Source: CAD feature listing. Evaluate the final solid. Frame: model axes, mm. A direction names the side the tool comes from. Round coordinates to 2 decimals unless told otherwise and drop trailing zeros. Loops run counter-clockwise (first coordinate to the right, second up) from the corner with the lowest first, then second, coordinate; pieces in that order, holes last. Notation, with made-up numbers: M 83,60.5 L 135,60.5 A7 cw 135,64.5 Z; hole C 32.25,42.5 d7. An arc over 180 degrees is marked long. One line per item, written item: value.
from build123d import *

# Parameters (mm, degrees)
BOSS_EXTRUDE1_DEPTH = 6.35


with BuildPart() as part:
    # Sketch1 → Boss-Extrude1 (new body)
    with BuildSketch(Plane(origin=(0, 0, 0), x_dir=(1, 0, 0), z_dir=(0, 1, 0))):
        with BuildLine():
            Line((71.346202472, -8.760212143), (83.951538598, -10.307952804))
            Line((83.951538598, -10.307952804), (83.177668268, -16.610620867))
            Line((83.177668268, -16.610620867), (89.48033633, -17.384491197))
            Line((89.48033633, -17.384491197), (90.254206661, -11.081823135))
            Line((90.254206661, -11.081823135), (96.556874724, -11.855693465))
            Line((96.556874724, -11.855693465), (97.231421537, -6.361950537))
            Line((97.231421537, -6.361950537), (95.20563486, -6.113215209))
            Line((95.20563486, -6.113215209), (95.559055961, -3.234831328))
            Line((95.559055961, -3.234831328), (97.584842638, -3.483566655))
            Line((97.584842638, -3.483566655), (98.259389451, 2.010176273))
            Line((98.259389451, 2.010176273), (102.545203734, 1.483944448))
            Line((102.545203734, 1.483944448), (101.870656921, -4.00979848))
            Line((101.870656921, -4.00979848), (103.896443599, -4.258533808))
            Line((103.896443599, -4.258533808), (103.543022498, -7.136917689))
            Line((103.543022498, -7.136917689), (101.51723582, -6.888182361))
            Line((101.51723582, -6.888182361), (100.842689007, -12.38192529))
            Line((100.842689007, -12.38192529), (107.14535707, -13.155795621))
            Line((107.14535707, -13.155795621), (106.371486739, -19.458463684))
            Line((106.371486739, -19.458463684), (112.674154802, -20.232334014))
            Line((112.674154802, -20.232334014), (113.448025133, -13.929665951))
            Line((113.448025133, -13.929665951), (115.769636124, 4.978338238))
            Line((115.769636124, 4.978338238), (44.17132693, 13.769505193))
            ThreePointArc((44.17132693, 13.769505193), (30.153869414, 53.312351607), (25.4, 94.996))
            Line((25.4, 94.996), (0, 94.996))
            Line((0, 94.996), (0, 0))
            Line((0, 0), (41.849715938, -5.138498995))
            Line((41.849715938, -5.138498995), (41.075845607, -11.441167058))
            Line((41.075845607, -11.441167058), (47.37851367, -12.215037389))
            Line((47.37851367, -12.215037389), (48.152384001, -5.912369326))
            Line((48.152384001, -5.912369326), (54.455052064, -6.686239657))
            Line((54.455052064, -6.686239657), (55.129598877, -1.192496728))
            Line((55.129598877, -1.192496728), (53.103812199, -0.9437614))
            Line((53.103812199, -0.9437614), (53.4572333, 1.934622481))
            Line((53.4572333, 1.934622481), (55.483019978, 1.685887153))
            Line((55.483019978, 1.685887153), (56.157566791, 7.179630082))
            Line((56.157566791, 7.179630082), (60.443381074, 6.653398257))
            Line((60.443381074, 6.653398257), (59.768834261, 1.159655329))
            Line((59.768834261, 1.159655329), (61.794620938, 0.910920001))
            Line((61.794620938, 0.910920001), (61.441199837, -1.967463881))
            Line((61.441199837, -1.967463881), (59.41541316, -1.718728553))
            Line((59.41541316, -1.718728553), (58.740866346, -7.212471481))
            Line((58.740866346, -7.212471481), (65.043534409, -7.986341812))
            Line((65.043534409, -7.986341812), (64.269664079, -14.289009875))
            Line((64.269664079, -14.289009875), (70.572332142, -15.062880206))
            Line((70.572332142, -15.062880206), (71.346202472, -8.760212143))
        make_face()
    extrude(amount=BOSS_EXTRUDE1_DEPTH)


solid = part.part
1. Ray query, line 1 (X direction, y = 2.25, z = -82.5); line 2 (X direction, y = 5.75, z = -85); line 3 (Z direction, x = 11.5, y = 5.25). Return the intervals inside material, ascending. Write a range as [from, to].
Report:
line 1: x = [0, 25.82]
line 2: x = [0, 25.67]
line 3: z = [-95, 1.41]
2. Section query B-B (x = 21). Return the cut outline in (y, z).
Report:
outline: M 0,-95 L 6.35,-95 L 6.35,2.58 L 0,2.58 Z
3. Section query A-A (z = -11.5). Return the cut outline in (x, y), and give its area (3 significant figures).
Report:
outline: M 0,0 L 62.65,0 L 62.65,6.35 L 0,6.35 Z
area: 398 mm2
4. Reachability of faces 4 (the face through (106.764, 3.131, 16.263)), 5 (the face through (41.468, 3.131, 8.246)), 6 (the face through (47.76, 3.13, 9.11)) from +Z, -Z, +X, -X, +Y, -Y: full face, straight path, thin tool, end or side. Return the list, or none.
Report:
face 4: +Y, -Y
face 5: -X, +Y, -Y
face 6: +Z, +Y, -Y
5. Pull-direction query (Z, two-part tool) for faces 1 (the face through (80.472, 3.131, -9.312)), 2 (the face through (95.38, 3.13, 4.69)), 3 (the face through (109.48, 3.13, 19.84)); classes: released by +Z, released by -Z, zero draft, split by the parting line, or undercut.
Report:
face 1: released by -Z
face 2: undercut
face 3: released by +Z
6. Pin query (flat end, axial travel): pin 1 (1.5 mm diameter, centred on x = 73, y = 5.5, fed in from -Z); pin 2 (1.5 mm diameter, centred on x = 51, y = 2, fed in from +Z); pin 3 (2 mm diameter, centred on y = 3.5, z = -28, fed in from +X). Return the tip coordinate at first contact, or that it passes through.
Report:
pin 1: stops at z = -10.32
pin 2: stops at z = 6.35
pin 3: stops at x = 38.34
